CAD build for the part. Positions are in the model's coordinates, mm. Round coordinates to 2 decimals unless told otherwise and drop trailing zeros. Loops run counter-clockwise (first coordinate to the right, second up) from the corner with the lowest first, then second, coordinate; pieces in that order, holes last. Notation, with made-up numbers: M 49.5,-37 L 67.5,-37 A19 ccw 67.5,-32 Z; hole C 70.25,-11 d5. An arc over 180 degrees is marked long. Use a Markdown table: item, result. Add a question column.
(1) Wall check: L1, parallel to Y at x = -16, z = 4.25; L2, parallel to Y at x = -45, z = 4.5; L3, parallel to X at y = 69, z = 1.25. Give the ranges that are in metal, low to high.
(2) Two-plate mould, pull along Y, no slides. Class faces 1 (the face through (-92.63, 94.65, 3.13)), 2 (the face through (-67, 0, 3)), 3 (the face through (-42.53, 88.61, 3.13)): released by +Y, released by -Y, zero draft, split by the parting line, or undercut.
(3) Band-saw the part on B-B, the plane y = 45. Write the cut outline in (x, z), and give its area (3 significant figures).
(4) Band-saw the part on C-C, the plane x = -16. Write the cut outline in (y, z).
(5) Flat gauge pins, fed straight in: P1, Ø7.5, axis at x = -44, y = 91.425, coming from the -Z side; P2, Ø4, axis at x = -16, y = 91.425, coming from the +Z side. Where does each tip first touch, or does it go through?
(6) Band-saw the part on D-D, the plane z = 2.75. Give the number of separate pieces and of enclosed holes in the cut face, and give its area (3 significant figures).
(7) Band-saw the part on A-A, the plane y = 68.15. Write the cut outline in (x, z) (3 decimals).
from build123d import *

# Parameters (mm, degrees)
CROQUIS1_R              = 3.175
SALIENTE_EXTRUIR1_DEPTH = 6.35
CROQUIS2_R              = 2.75
CROQUIS2_R_2            = 17.4625
CORTAR_EXTRUIR1_DEPTH   = 12.7


with BuildPart() as part:
    # Croquis1 → Saliente-Extruir1 (new body)
    with BuildSketch(Plane.XY):
        Polygon((0, 0), (-135, 0), (-135, 70), (-49.056075443, 120), (0, 120), align=None)
        with Locations((-44, 110.475)):
            Circle(CROQUIS1_R, mode=Mode.SUBTRACT)
        with Locations((-16, 110.475)):
            Circle(CROQUIS1_R, mode=Mode.SUBTRACT)
        with Locations((-16, 91.425)):
            Circle(CROQUIS1_R, mode=Mode.SUBTRACT)
        with Locations((-44, 91.425)):
            Circle(CROQUIS1_R, mode=Mode.SUBTRACT)
    extrude(amount=SALIENTE_EXTRUIR1_DEPTH)

    # Croquis2 → Cortar-Extruir1 (cut)
    with BuildSketch(Plane.XY.offset(6.35)):
        with Locations((-128.145, 68.15)):
            Circle(CROQUIS2_R)
        with Locations((-128.145, 21.85)):
            Circle(CROQUIS2_R)
        with Locations((-81.855, 21.85)):
            Circle(CROQUIS2_R)
        with Locations((-81.855, 68.15)):
            Circle(CROQUIS2_R)
        with Locations((-105, 45)):
            Circle(CROQUIS2_R_2)
    extrude(amount=-CORTAR_EXTRUIR1_DEPTH, mode=Mode.SUBTRACT)


solid = part.part
Return value:
| question | item | result |
|---|---|---|
| 1 | L1 | 0 to 88.25, 94.6 to 107.3, 113.65 to 120 |
| 1 | L2 | 0 to 88.41, 94.44 to 107.46, 113.49 to 120 |
| 1 | L3 | -135 to -130.76, -125.53 to -84.47, -79.24 to 0 |
| 2 | face 1 | released by +Y |
| 2 | face 2 | released by -Y |
| 2 | face 3 | undercut |
| 3 | outline | M -135,0 L -122.46,0 L -122.46,6.35 L -135,6.35 Z; M -87.54,0 L 0,0 L 0,6.35 L -87.54,6.35 Z |
| 3 | area | 635 mm^2 |
| 4 | outline | M 0,0 L 88.25,0 L 88.25,6.35 L 0,6.35 Z; M 94.6,0 L 107.3,0 L 107.3,6.35 L 94.6,6.35 Z; M 113.65,0 L 120,0 L 120,6.35 L 113.65,6.35 Z |
| 5 | P1 | z = 0 |
| 5 | P2 | through |
| 6 | separate pieces | 1 |
| 6 | enclosed holes | 9 |
| 6 | area | 12,900 mm^2 |
| 7 | outline | M -135,0 L -130.895,0 L -130.895,6.35 L -135,6.35 Z; M -125.395,0 L -84.605,0 L -84.605,6.35 L -125.395,6.35 Z; M -79.105,0 L 0,0 L 0,6.35 L -79.105,6.35 Z |
